CAD build for the part. Positions are in the model's coordinates, mm. Face numbers are marked on the shaded views. A direction names the side the tool comes from. Give positions to 0.01 mm unless a question says otherwise; leave off trailing zeros. Write each loop counter-clockwise with the first axis right and the second up, starting at its lowest first coordinate (ties: lowest second). Pieces come first, ordered by that corner, then holes. Notation, with made-up numbers: (77.5, 9) -> (86.5, 9) arc R23 cw to (86.5, 47) -> close; hole circle Ø1 at (66.5, -18). An arc over 180 degrees is marked (long way). Answer in a Markdown table with one row per item. Add a question column.
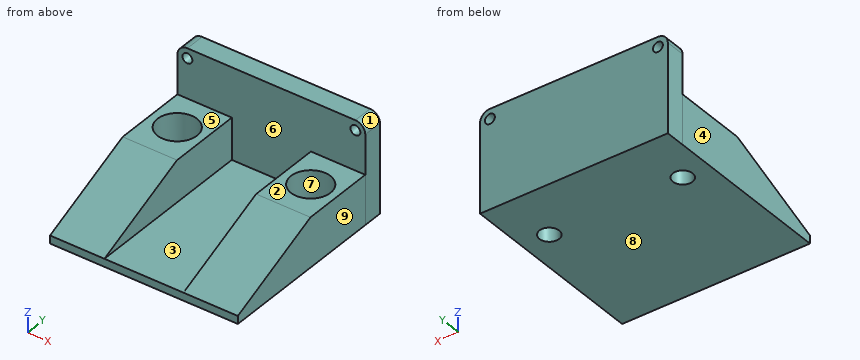
```python
from build123d import *

# Parameters (mm, degrees)
F0_W            = 40
F0_H            = 86.76
F1_DEPTH        = 4
F2_W            = 95
F2_H            = 25
F3_DEPTH        = 27.5
F4_W            = 86.76
F4_H            = 25
F5_DEPTH        = 27.5
F6_W            = 94.977141
F6_H            = 50
F7_DEPTH        = 10
F9_R            = 5
F10_R           = 5
F11_R           = 2.5
F12_DEPTH       = 10.001
F14_DEPTH       = 95.001
F16_D           = 10
F16_CBORE_D     = 20
F16_CBORE_DEPTH = 15
F17_D           = 10
F17_CBORE_D     = 20
F17_CBORE_DEPTH = 15


with BuildPart() as f1:
    # F0 (on Top) → F1 (new body)
    with BuildSketch(Plane.XY):
        Rectangle(F0_W, F0_H)
    extrude(amount=F1_DEPTH)

    # F2 (on face) → F3 (join)
    with BuildSketch(Plane.YZ.offset(20)):
        with Locations((4.12, 12.5)):
            Rectangle(F2_W, F2_H)
    extrude(amount=F3_DEPTH)

    # F4 (on face) → F5 (join)
    with BuildSketch(Plane(origin=(-20, 0, 0), x_dir=(0, -1, 0), z_dir=(-1, 0, 0))):
        with Locations((0, 12.5)):
            Rectangle(F4_W, F4_H)
    extrude(amount=F5_DEPTH)

    # F6 (on face) → F7 (join)
    with BuildSketch(Plane(origin=(0, 43.38, 0), x_dir=(-1, 0, 0), z_dir=(0, 1, 0))):
        with Locations((-0.01143, 25)):
            Rectangle(F6_W, F6_H)
    extrude(amount=F7_DEPTH)

    # F9
    f9_edges = [f1.edges().sort_by_distance(p)[0] for p in [
        (47.5, 48.38, 50),
    ]]
    fillet(f9_edges, radius=F9_R)

    # F10
    f10_edges = [f1.edges().sort_by_distance(p)[0] for p in [
        (-47.477141, 48.38, 50),
    ]]
    fillet(f10_edges, radius=F10_R)

    # F11 (on face) → F12 (cut, through all)
    with BuildSketch(Plane.XZ.offset(-43.38)):
        with Locations((-42.477141, 45)):
            Circle(F11_R)
        with Locations((42.5, 45)):
            Circle(F11_R)
    extrude(amount=-F12_DEPTH, mode=Mode.SUBTRACT)

    # F13 (on face) → F14 (cut, through all)
    with BuildSketch(Plane(origin=(-47.5, 0, 0), x_dir=(0, -1, 0), z_dir=(-1, 0, 0))):
        Polygon((43.38, 25), (-6.08, 25), (43.38, 4), align=None)
    extrude(amount=-F14_DEPTH, mode=Mode.SUBTRACT)

    # F16 (through all)
    with Locations(Plane.XY.offset(25)):
        with Locations((-33.75, 24.73)):
            CounterBoreHole(F16_D / 2, F16_CBORE_D / 2, F16_CBORE_DEPTH)

    # F17 (through all)
    with Locations(Plane.XY.offset(25)):
        with Locations((33.75, 24.73)):
            CounterBoreHole(F17_D / 2, F17_CBORE_D / 2, F17_CBORE_DEPTH)


solid = f1.part
```
Item 1: Slice it at A-A, the plane y = 24.73. List the corners of the cut face in (x, z).
Item 2: Slice it at D-D, the plane x = -7.5. List the corners of the cut face in (y, z), then the cut area to 3 significant figures.
Item 3: Probe L1, parallel to X at y = -10, z = 5; L2, parallel to Y at x = 33.75, z = 21.25; L3, parallel to Y at x = 40, z = 43.5. List the from-to ranges inside material, lowest first. Write a range as from..to.
Item 4: Which spindle directions (+Z, -Z, +X, -X, +Y, -Y) get a long thin tool onto all of the face, cutting with end or side? Do the marked faces 5, 6, 7, 8 and 9. Say none if no direction does.
Item 5: Mould opens along X. For the marked faces 1, 2, 3 and 4 say: released by +X, released by -X, zero draft, split by the parting line, or undercut.
Item 6: Slice it at B-B, the plane x = -33.75. List the corners of the cut face in (y, z).
Item 7: Slice it at C-C, the plane z = 7.5. State how many separate pieces and enclosed holes the cut face has, then the cut area to 3 significant figures.
Item 8: Drop flat-ended pins along their axis: pin 1 Ø8 at (x, y) = (33.75, 24.73) entering from +Z; pin 2 Ø6 at (x, y) = (-24.5, -12) entering from +Z; pin 3 Ø2 at (x, y) = (-10, -28) entering from +Z; pin 4 Ø22 at (x, y) = (31, 22.5) entering from +Z. Give the stop position or say it passes through.
Answer key:
| question | item | result |
|---|---|---|
| 1 | outline | (-47.5, 0) -> (-38.75, 0) -> (-38.75, 10) -> (-43.75, 10) -> (-43.75, 25) -> (-47.5, 25) -> close; (-28.75, 0) -> (28.75, 0) -> (28.75, 10) -> (23.75, 10) -> (23.75, 25) -> (20, 25) -> (20, 4) -> (-20, 4) -> (-20, 25) -> (-23.75, 25) -> (-23.75, 10) -> (-28.75, 10) -> close; (38.75, 0) -> (47.5, 0) -> (47.5, 25) -> (43.75, 25) -> (43.75, 10) -> (38.75, 10) -> close |
| 2 | outline | (-43.38, 0) -> (53.38, 0) -> (53.38, 50) -> (43.38, 50) -> (43.38, 4) -> (-43.38, 4) -> close |
| 2 | area | 847 mm² |
| 3 | L1 | x = -47.5..-20, 20..47.5 |
| 3 | L2 | y = -2.75..14.73, 34.73..53.38 |
| 3 | L3 | y = 43.38..53.38 |
| 4 | face 5 | +Z, +X, -X, -Y |
| 4 | face 6 | +Z, -Y |
| 4 | face 7 | +Z |
| 4 | face 8 | -Z, +X, -X, +Y, -Y |
| 4 | face 9 | +Z, -Z, +X, +Y, -Y |
| 5 | face 1 | released by +X |
| 5 | face 2 | zero draft |
| 5 | face 3 | undercut |
| 5 | face 4 | released by -X |
| 6 | outline | (-43.38, 0) -> (19.73, 0) -> (19.73, 10) -> (14.73, 10) -> (14.73, 25) -> (6.08, 25) -> (-43.38, 4) -> close; (29.73, 0) -> (53.38, 0) -> (53.38, 50) -> (43.38, 50) -> (43.38, 25) -> (34.73, 25) -> (34.73, 10) -> (29.73, 10) -> close |
| 7 | separate pieces | 1 |
| 7 | enclosed holes | 2 |
| 7 | area | 5,110 mm² |
| 8 | pin 1 | passes through |
| 8 | pin 2 | stops at z = 18.6 |
| 8 | pin 3 | stops at z = 4 |
| 8 | pin 4 | stops at z = 25 |
